Model file for the job. Use its own axes, mm. A direction names the side the tool comes from. Round coordinates to 2 decimals unless told otherwise and drop trailing zeros. Order: outer loops, then holes, each group sorted by start corner. A loop starts at its lowest first (then second) coordinate and runs counter-clockwise, first axis right, second up. Notation, with made-up numbers: (30, 2.25) -> (36, 2.25) arc R25 cw to (36, 16.25) -> close; hole circle Ø7 at (-35.5, 9.25). An arc over 180 degrees is marked (long way). Put each result on its own line as item: value. Start each with the question number.
Q1. Cut at B-B, the plane y = -2. List the corners of the cut face in (x, z), and give its area (3 significant figures).
Q2. Probe L1, parallel to X at y = 4, z = 9; L2, parallel to X at y = 4, z = 6.55; L3, parallel to Z at x = 194.5, y = 0. List the from-to ranges inside material, lowest first.
Q3. Pull direction Y, two halves, no side cores. Call faces 5 (the face through (148, -10, 14)), 6 (the face through (300, -5, 9)), 7 (the face through (277.883, 5.5, 6.507)), 8 (the face through (26.4, 5.4, 7)): released by +Y, released by -Y, zero draft, split by the parting line, or undercut.
Q4. Cut at C-C, the plane z = 13. List the corners of the cut face in (x, y), and give its area (3 significant figures).
Q5. Flat gauge pins, fed straight in: P1, Ø4.5, axis at x = 111, z = 19.5, coming from the +Y side; P2, Ø2, axis at x = 24.5, y = 5.5, coming from the -Z side; P3, Ø2, axis at x = 150, y = 4, coming from the -Z side; P4, Ø10, axis at x = 132.5, y = 6, coming from the +Z side. Where does each tip first touch, or does it go through?
Q6. Cut at A-A, the plane x = 43.5. List the corners of the cut face in (y, z), and give its area (3 significant figures).
Q7. 3-axis set-ups, long thin cutter, end or side, ignore diameter. For faces 1 (the face through (148, -13, 27)), 2 (the face through (148, -10, 26)), 3 (the face through (148, 4, 10)), 4 (the face through (276.4, 5.4, 7)): which of +Z, -Z, +X, -X, +Y, -Y reach the whole face in a straight line?
Autodesk Inventor part; units mm, degrees
ref_plane "YZ Plane" through (0, 0, 0) normal (1, 0, 0) x (0, 1, 0)
ref_plane "XZ Plane" through (0, 0, 0) normal (0, 1, 0) x (-1, 0, 0)
ref_plane "XY Plane" through (0, 0, 0) normal (0, 0, 1) x (1, 0, 0)
sketch "Sketch1" plane through (0, 0, 0) normal (1, 0, 0) x (0, 1, 0)
  line L0 (0, 0) -> (4, 0)
  line L1 (4, 0) -> (4, 20)
  line L2 (4, 20) -> (0, 20) construction
  line L3 (0, 20) -> (0, 0)
  line L4 (4, 20) -> (12, 28)
  line L5 (12, 28) -> (16, 28)
  line L6 (16, 28) -> (24, 20)
  line L7 (24, 20) -> (24, 24)
  line L8 (24, 24) -> (17.1716, 30.8284)
  line L9 (17.1716, 30.8284) -> (10.8284, 30.8284)
  line L10 (10.8284, 30.8284) -> (0, 20)
  line L11 (24, 20) -> (4, 20) construction
  line L12 (14, 30.8284) -> (14, 28) construction
  dimension "d0" = 20
  dimension "d1" = 4
  dimension "d8" = 135
  dimension "d11" = 20
  dimension "d12" = 8
  dimension "d13" = 2.8284
  dimension "d14" = 2.8284
extrude "Extrusion1" add sketch "Sketch1" along normal blind 300
sketch "Sketch2" plane through (0, 0, 0) normal (0, -1, 0) x (1, 0, 0)
  line L0 (300, 0) -> (300, 20)
  line L1 (300, 10) -> (275, 10)
  line L2 (275, 10) -> (150, 10)
  line L3 (150, 10) -> (25, 10)
  line L4 (25, 10) -> (0, 10)
  line L5 (0, 0) -> (300, 0)
  line L6 (0, 20) -> (0, 0)
  dimension "d15" = 10
  dimension "d16" = 25
hole "Hole1" at (275, 0, 10) at (150, 0, 10) at (25, 0, 10) direction (0, 1, 0) diameter 3.4 end through all counterbore diameter 6.5 counterbore depth 1
move or copy body "Rotate1" bodies to move or copy 1 copy no rotation origin (0, 0, 0) rotation axis (1, 0, 0) rotation angle 90 translate (0, 14, 6)
equation "\"d13\" = d14"
properties part number "Rear_Rail_Wire_Cover"
Ans:
1. outline: (0, 6) -> (300, 6) -> (300, 10) -> (0, 10) -> close
1. area: 1,200 mm^2
2. L1: x = 0 to 23.3, 26.7 to 148.3, 151.7 to 273.3, 276.7 to 300
2. L2: x = 0 to 21.75, 28.25 to 146.75, 153.25 to 271.75, 278.25 to 300
2. L3: z = 6 to 10
3. face 5: released by +Y
3. face 6: zero draft
3. face 7: undercut
3. face 8: undercut
4. outline: (0, -13) -> (300, -13) -> (300, -9) -> (0, -9) -> close
4. area: 1,200 mm^2
5. P1: stops at y = -13.25
5. P2: stops at z = 7
5. P3: passes through
5. P4: stops at z = 10
6. outline: (-16.83, 16.83) -> (-6, 6) -> (14, 6) -> (14, 10) -> (-6, 10) -> (-14, 18) -> (-14, 22) -> (-6, 30) -> (-10, 30) -> (-16.83, 23.17) -> close
6. area: 162 mm^2
7. face 1: +Z, +X, -X, -Y
7. face 2: +X, -X, +Y
7. face 3: +Z, +X, -X, +Y
7. face 4: -Z
